from build123d import *

# Parameters (mm, degrees)
SKETCH1_R             = 4.445
SKETCH1_R_2           = 6.477
SKETCH1_R_3           = 2.19075
BOSS_EXTRUDE1_DEPTH   = 6.35
F_1_0MM_DOWEL_HOLE2_D = 3.0226


with BuildPart() as part:
    # Sketch1 → Boss-Extrude1 (new body)
    with BuildSketch(Plane.XZ):
        with BuildLine():
            Line((-35.56, -19.05), (111.76, -19.05))
            ThreePointArc((111.76, -19.05), (113.556051224, -18.306051224), (114.3, -16.51))
            Line((114.3, -16.51), (114.3, 16.51))
            ThreePointArc((114.3, 16.51), (113.556051224, 18.306051224), (111.76, 19.05))
            Line((111.76, 19.05), (-35.56, 19.05))
            ThreePointArc((-35.56, 19.05), (-37.356051224, 18.306051224), (-38.1, 16.51))
            Line((-38.1, 16.51), (-38.1, -16.51))
            ThreePointArc((-38.1, -16.51), (-37.356051224, -18.306051224), (-35.56, -19.05))
        make_face()
        with Locations(Location((59.69, 0, 0), (0, 0, 270))):
            Circle(SKETCH1_R, mode=Mode.SUBTRACT)
        with Locations(Location((97.79, 0, 0), (0, 0, 270))):
            Circle(SKETCH1_R, mode=Mode.SUBTRACT)
        with Locations(Location((-21.59, 0, 0), (0, 0, 270))):
            Circle(SKETCH1_R_2, mode=Mode.SUBTRACT)
        with Locations(Location((-21.59, -10.31875, 0), (0, 0, 270))):
            Circle(SKETCH1_R_3, mode=Mode.SUBTRACT)
        with Locations(Location((-21.59, 10.31875, 0), (0, 0, 270))):
            Circle(SKETCH1_R_3, mode=Mode.SUBTRACT)
        with Locations(Location((21.59, 0, 0), (0, 0, 90))):
            Circle(SKETCH1_R, mode=Mode.SUBTRACT)
    extrude(amount=-BOSS_EXTRUDE1_DEPTH)

    # Ø1.0mm Dowel Hole2 (through all)
    with Locations(Plane(origin=(0, 6.35, 0), x_dir=(1, 0, 0), z_dir=(0, 1, 0))):
        with Locations((-34.29, 15.24), (110.49, 15.24), (110.49, -15.24), (-34.29, -15.24)):
            Hole(F_1_0MM_DOWEL_HOLE2_D / 2)


solid = part.part
Work out the finished part from the listing and answer in its coordinate system (mm). Coordinates: 2 decimals unless noted, no trailing zeros. Order: outer loops, then holes, each group sorted by start corner. A loop starts at its lowest first (then second) coordinate and runs counter-clockwise, first axis right, second up. Notation, with made-up numbers: (28.5, 51) - (43.5, 51) arc R24 ccw to (43.5, 77) - close; hole circle Ø9 at (9, 11.25). An arc over 180 degrees is marked (long way). Put each result on its own line as item: value. Start each with the question number.
1) Find section C-C (y = 1.5). State how many separate pieces and enclosed holes the cut face has, plus the area to 3 significant figures.
2) For a pull along X with two mould halves and no side action, classify faces 1 (the cylindrical face through (-37.336, 3.131, 18.326)), 2 (the flat face through (114.3, 3, 0)), 3 (the flat face through (37, 3, -19.05)), 4 (the cylindrical face through (25.93, 3.13, -0.96)) as released by +X, released by -X, zero draft, split by the parting line, or undercut.
3) Find section A-A (z = 0). Give the vertices of the cut face in (x, y) (3 decimals), plus the area to 3 significant figures.
4) Find section D-D (x = -34.29). Give the vertices of the cut face in (y, z).
5) Find the intervals of material crossed by line 1 (X direction, y = 6.25, z = -15); line 2 (X direction, y = 4.25, z = 0) (3 decimals); line 3 (Z direction, x = 110.49, y = 3.75), in increasing order. Write a range as from..to.
6) Find section B-B (x = 97.79). Give the vertices of the cut face in (y, z) (3 decimals), plus the area to 3 significant figures.
Results list:
1. separate pieces: 1
1. enclosed holes: 10
1. area: 5,420 mm^2
2. face 1: released by -X
2. face 2: released by +X
2. face 3: zero draft
2. face 4: undercut
3. outline: (-38.1, 0) - (-28.067, 0) - (-28.067, 6.35) - (-38.1, 6.35) - close; (-15.113, 0) - (17.145, 0) - (17.145, 6.35) - (-15.113, 6.35) - close; (26.035, 0) - (55.245, 0) - (55.245, 6.35) - (26.035, 6.35) - close; (64.135, 0) - (93.345, 0) - (93.345, 6.35) - (64.135, 6.35) - close; (102.235, 0) - (114.3, 0) - (114.3, 6.35) - (102.235, 6.35) - close
3. area: 716 mm^2
4. outline: (0, -19.05) - (6.35, -19.05) - (6.35, -16.75) - (0, -16.75) - close; (0, -13.73) - (6.35, -13.73) - (6.35, 13.73) - (0, 13.73) - close; (0, 16.75) - (6.35, 16.75) - (6.35, 19.05) - (0, 19.05) - close
5. line 1: x = -38.1..-35.78, -32.8..109, 111.98..114.3
5. line 2: x = -38.1..-28.067, -15.113..17.145, 26.035..55.245, 64.135..93.345, 102.235..114.3
5. line 3: z = -19.05..-16.75, -13.73..13.73, 16.75..19.05
6. outline: (0, -19.05) - (6.35, -19.05) - (6.35, -4.445) - (0, -4.445) - close; (0, 4.445) - (6.35, 4.445) - (6.35, 19.05) - (0, 19.05) - close
6. area: 185 mm^2
